```python
from build123d import *

# Parameters (mm, degrees)
BOSS_EXTRUDE1_DEPTH = 3.175
SKETCH2_W           = 3.175
SKETCH2_H           = 178.054
BOSS_EXTRUDE2_DEPTH = 11.303


with BuildPart() as part:
    # Sketch1 → Boss-Extrude1 (new body)
    with BuildSketch(Plane(origin=(0, 0, 0), x_dir=(0, 0, -1), z_dir=(1, 0, 0))):
        with BuildLine():
            Line((0, 0), (178.054, 0))
            ThreePointArc((178.054, 0), (164.500446282, 68.138315866), (125.903190817, 125.903190817))
            Line((125.903190817, 125.903190817), (0, 0))
        make_face()
    extrude(amount=BOSS_EXTRUDE1_DEPTH)

    # Sketch2 → Boss-Extrude2 (add)
    with BuildSketch(Plane.XZ):
        with Locations((1.5875, -89.027)):
            Rectangle(SKETCH2_W, SKETCH2_H)
    extrude(amount=BOSS_EXTRUDE2_DEPTH)


solid = part.part
```
Part model, mm, in its own coordinate system. Round coordinates to 2 decimals unless told otherwise and drop trailing zeros. Loops run counter-clockwise (first coordinate to the right, second up) from the corner with the lowest first, then second, coordinate; pieces in that order, holes last. Notation, with made-up numbers: (70, -32.5) -> (113, -32.5) arc R27 ccw to (113, 4.5) -> close; hole circle Ø11 at (33, -6.75). An arc over 180 degrees is marked (long way). Use CSV: the item, a comma, the result in double quotes. Start each with the question number.
1) Wall check: L1, parallel to Y at x = 1.45, z = -109; L2, parallel to Y at x = 2, z = -136; L3, parallel to Z at x = 1.1, y = 101. Give the ranges that are in metal, low to high. Write a range as [from, to].
2) Drop flat-ended pins along their axis: P1, Ø1.5, axis at x = 0.5, y = 81.5, coming from the +Z side; P2, Ø1, axis at x = 1, y = 61, coming from the -Z side; P3, Ø1, axis at x = 1, z = -111, coming from the +Y side. Give the stop position or say it passes through.
3) Cut at B-B, the plane z = -83. Write the cut outline in (x, y) (3 decimals), plus the area to 3 significant figures.
4) Cut at C-C, the plane y = 24. Write the cut outline in (x, z) (3 decimals).
5) Cut at A-A, the plane x = 2.65. Write the cut outline in (y, z), plus the area to 3 significant figures.
Determined:
1,L1,"y = [-11.3, 109]"
1,L2,"y = [-11.3, 114.92]"
1,L3,"z = [-146.64, -101]"
2,P1,"stops at z = -80.75"
2,P2,"stops at z = -167.46"
2,P3,"stops at y = 111.5"
3,outline,"(0, -11.303) -> (3.175, -11.303) -> (3.175, 83) -> (0, 83) -> close"
3,area,"299 mm2"
4,outline,"(0, -176.429) -> (3.175, -176.429) -> (3.175, -24) -> (0, -24) -> close"
5,outline,"(-11.3, -178.05) -> (0, -178.05) arc R178.05 ccw to (125.9, -125.9) -> (0, 0) -> (-11.3, 0) -> close"
5,area,"14,500 mm2"
